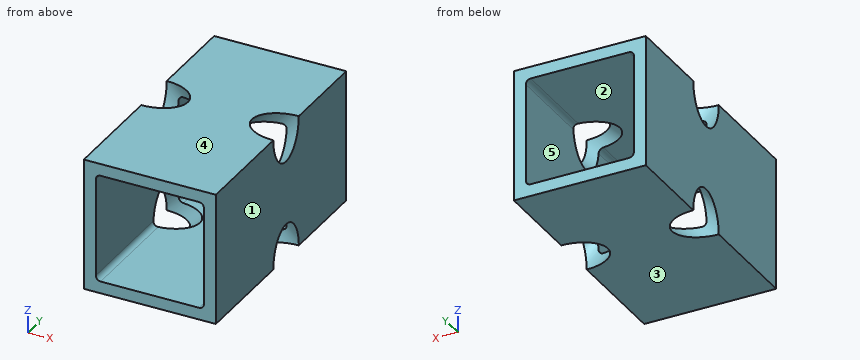
```python
from build123d import *

# Parameters (mm, degrees)
SKETCH1_W               = 34.925
SKETCH1_H               = 34.925
SKETCH1_W_2             = 28.575
SKETCH1_H_2             = 28.575
BOSS_EXTRUDE1_DEPTH     = 65
FILLET1_R               = 1.27
SKETCH2_R               = 6.35
CUT_EXTRUDE1_DEPTH      = 25.695704333
CUT_EXTRUDE1_DEPTH_BACK = 25.695704333
SKETCH3_R               = 6.35
CUT_EXTRUDE2_DEPTH      = 25.695704474
CUT_EXTRUDE2_DEPTH_BACK = 25.695704474


with BuildPart() as part:
    # Sketch1 → Boss-Extrude1 (new body)
    with BuildSketch(Plane(origin=(0, 0, 0), x_dir=(1, 0, 0), z_dir=(0, 1, 0))):
        Rectangle(SKETCH1_W, SKETCH1_H)
        Rectangle(SKETCH1_W_2, SKETCH1_H_2, mode=Mode.SUBTRACT)
    extrude(amount=BOSS_EXTRUDE1_DEPTH)

    # Fillet1
    fillet1_edges = [part.edges().sort_by_distance(p)[0] for p in [
        (-14.2875, 32.5, 14.2875),
        (14.2875, 32.5, 14.2875),
        (14.2875, 32.5, -14.2875),
        (-14.2875, 32.5, -14.2875),
    ]]
    fillet(fillet1_edges, radius=FILLET1_R)

    # Sketch2 → Cut-Extrude1 (cut, two sides)
    with BuildSketch(Plane(origin=(0, 0, 0), x_dir=(0.707106781, 0, 0.707106781), z_dir=(-0.707106781, 0, 0.707106781))) as cut_extrude1_sk:
        with Locations((0, 35)):
            Circle(SKETCH2_R)
    extrude(amount=CUT_EXTRUDE1_DEPTH, mode=Mode.SUBTRACT)
    extrude(cut_extrude1_sk.sketch, amount=-CUT_EXTRUDE1_DEPTH_BACK, mode=Mode.SUBTRACT)

    # Sketch3 → Cut-Extrude2 (cut, two sides)
    with BuildSketch(Plane(origin=(0, 0, 0), x_dir=(0.707106781, 0, -0.707106781), z_dir=(0.707106781, 0, 0.707106781))) as cut_extrude2_sk:
        with Locations((0, 35)):
            Circle(SKETCH3_R)
    extrude(amount=CUT_EXTRUDE2_DEPTH, mode=Mode.SUBTRACT)
    extrude(cut_extrude2_sk.sketch, amount=-CUT_EXTRUDE2_DEPTH_BACK, mode=Mode.SUBTRACT)


solid = part.part
```
Geometry check sheet. Reference: the model listing, model coordinates, mm. Face numbers are marked on the shaded views. A direction names the side the tool comes from. Coordinates: 2 decimals unless noted, no trailing zeros. Order: outer loops, then holes, each group sorted by start corner. A loop starts at its lowest first (then second) coordinate and runs counter-clockwise, first axis right, second up.
Item 1: Tool access check on the marked faces 1 and 2. Record the directions out of +Z, -Z, +X, -X, +Y, -Y that give a thin tool (end or side, any length) a straight path to the whole face; none if there is none.
Item 2: Section check B-B (x = 0). Enter the section's corners in (y, z), plus the area to 3 significant figures.
Item 3: Scan lines: line 1 along Z through (x, y) = (-9.5, 7.5); line 2 along Z through (x, y) = (13.5, 46). Record each from-to range of solid material in increasing order.
Item 4: Section check D-D (z = -12). Count the separate pieces of the cut face and the enclosed holes in it, plus the area to 3 significant figures.
Item 5: Mould release check, pull along Z, two halves, no side actions. Record for the marked faces 3, 4 and 5: released by +Z, released by -Z, zero draft, split by the parting line, or undercut.
Item 6: Section check A-A (z = 2). Enter the section's corners in (x, y), plus the area to 3 significant figures.
Item 7: Section check C-C (y = 9). Enter the section's corners in (x, z).
Check sheet entries:
1. face 1: +Z, -Z, +X, +Y, -Y
1. face 2: +Y, -Y
2. outline: (0, -17.46) - (65, -17.46) - (65, -14.29) - (0, -14.29) - close; (0, 14.29) - (65, 14.29) - (65, 17.46) - (0, 17.46) - close
2. area: 413 mm2
3. line 1: z = -17.46 to -14.29, 14.29 to 17.46
3. line 2: z = -17.46 to -14.19, 14.19 to 17.46
4. separate pieces: 4
4. enclosed holes: 0
4. area: 341 mm2
5. face 3: released by -Z
5. face 4: released by +Z
5. face 5: undercut
6. outline: (-17.46, 0) - (-14.29, 0) - (-14.29, 65) - (-17.46, 65) - close; (14.29, 0) - (17.46, 0) - (17.46, 65) - (14.29, 65) - close
6. area: 413 mm2
7. outline: (-17.46, -17.46) - (17.46, -17.46) - (17.46, 17.46) - (-17.46, 17.46) - close; hole (-14.29, -13.02) arc R1.27 ccw to (-13.02, -14.29) - (13.02, -14.29) arc R1.27 ccw to (14.29, -13.02) - (14.29, 13.02) arc R1.27 ccw to (13.02, 14.29) - (-13.02, 14.29) arc R1.27 ccw to (-14.29, 13.02) - close
